```python
from build123d import *

# Parameters (mm, degrees)
F0_W     = 76.2
F0_H     = 76.2
F1_DEPTH = 76.2
F3_D     = 25.4
F4_W     = 25.4
F4_H     = 25.4
F5_DEPTH = 12.7
F6_R     = 12.7
F7_DEPTH = 12.7
F9_DEPTH = 152.4


with BuildPart() as f1:
    # F0 (on Front) → F1 (new body)
    with BuildSketch(Plane.XZ):
        with Locations((11.565426, 19.49024)):
            Rectangle(F0_W, F0_H)
    extrude(amount=F1_DEPTH)

    # F3 (through all)
    with Locations(Plane.XY.offset(57.59024)):
        with Locations((11.565426, -38.1)):
            Hole(F3_D / 2)

    # F4 (on face) → F5 (join)
    with BuildSketch(Plane(origin=(-26.534574, 0, 0), x_dir=(0, -1, 0), z_dir=(-1, 0, 0))):
        with Locations((38.1, 19.49024)):
            Rectangle(F4_W, F4_H)
    extrude(amount=F5_DEPTH)

    # F6 (on face) → F7 (join)
    with BuildSketch(Plane.XZ.offset(76.2)):
        with Locations((11.565426, 19.49024)):
            Circle(F6_R)
    extrude(amount=F7_DEPTH)

    # F8 (on face) → F9 (join)
    with BuildSketch(Plane(origin=(0, 0, 0), x_dir=(-1, 0, 0), z_dir=(0, 1, 0))):
        Polygon((0.204802, 37.538857), (-36.691747, 13.577958), (2.507274, -6.394941), align=None)
    extrude(amount=F9_DEPTH)


solid = f1.part
```
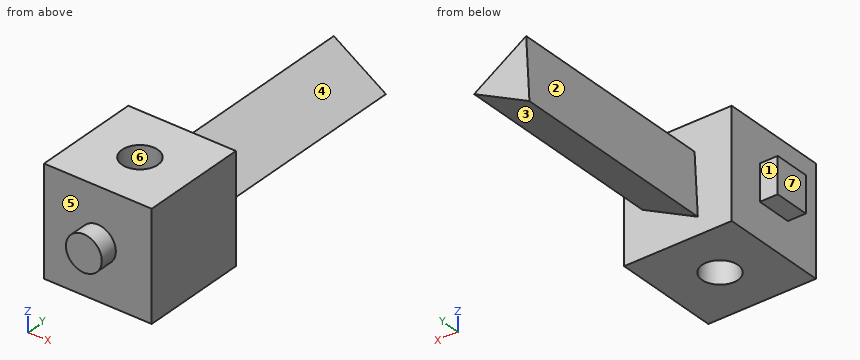
Could you check a few things on this model? Use its own coordinates, in mm. Face numbers are marked on the shaded views. A direction names the side the tool comes from. Round coordinates to 2 decimals unless told otherwise and drop trailing zeros. Write each loop counter-clockwise with the first axis right and the second up, starting at its lowest first coordinate (ties: lowest second). Pieces come first, ordered by that corner, then holes. Notation, with made-up numbers: M 13.5,-17 L 61.5,-17 A34 cw 61.5,19 Z; hole C 0,36 d9. An arc over 180 degrees is marked long. Answer in a Markdown table with one row per item. Add a question column.
Q1. If I drill on line 1 (X direction, y = -38, z = 0); line 2 (Y direction, x = -31.5, z = 12.5); line 3 (Y direction, x = -21, z = 26), over which ranges is the centre line in solid material (lowest first)? Write a range as from..to.
Q2. If we mould it in two halves opening along X, with no side actions, what happens to the marked faces 4, 5, 6 and 7? For each: +X half, -X half, draft (parallel to the pull), parting line (faces both ways), or undercut.
Q3. Imagine slicing it at D-D (y = 14). Please give me the cut outline in (x, z).
Q4. On a 3-axis mill with a long thin cutter (end or side, diameter ignored), from which of +Z, -Z, +X, -X, +Y, -Y can I reach the whole of each face in a straight line? I mean the marked faces 1, 2 and 3. Say none if no direction works.
Q5. Imagine slicing it at B-B (z = -10.5). Please give me the cut outline in (x, y), then the cut area to 3 significant figures.
Q6. Imagine slicing it at A-A (y = -38.1). Please give me the cut outline in (x, z).
Q7. Will these pins go through, and if not, where does the flat tip stop? pin 1 Ø6.5 at (x, y) = (-34, -38) entering from +Z; pin 2 Ø5 at (y, z) = (-6.5, -9) entering from -X; pin 3 Ø4 at (x, z) = (-32, 18.5) entering from -Y; pin 4 Ø10 at (x, y) = (-30.5, -40.5) entering from -Z.
Q8. Imagine slicing it at C-C (x = 42.5). Please give me the cut outline in (y, z), then the cut area to 3 significant figures.
Values:
| question | item | result |
|---|---|---|
| 1 | line 1 | -26.53..-1.13, 24.27..49.67 |
| 1 | line 2 | -50.8..-25.4 |
| 1 | line 3 | -76.2..0 |
| 2 | face 4 | +X half |
| 2 | face 5 | draft |
| 2 | face 6 | undercut |
| 2 | face 7 | -X half |
| 3 | outline | M -2.51,-6.39 L 36.69,13.58 L -0.2,37.54 Z |
| 4 | face 1 | +Z, -Z, -X, +Y |
| 4 | face 2 | +Z, -X, +Y |
| 4 | face 3 | -Z, +X, +Y |
| 5 | outline | M -26.53,-76.2 L 49.67,-76.2 L 49.67,0 L -26.53,0 Z; hole C 11.57,-38.1 d25.4 |
| 5 | area | 5,300 mm^2 |
| 6 | outline | M -39.23,6.79 L -26.53,6.79 L -26.53,-18.61 L -1.13,-18.61 L -1.13,57.59 L -26.53,57.59 L -26.53,32.19 L -39.23,32.19 Z; M 24.27,-18.61 L 49.67,-18.61 L 49.67,57.59 L 24.27,57.59 Z |
| 7 | pin 1 | z = 32.19 |
| 7 | pin 2 | x = -26.53 |
| 7 | pin 3 | y = -50.8 |
| 7 | pin 4 | z = -18.61 |
| 8 | outline | M -76.2,-18.61 L 0,-18.61 L 0,57.59 L -76.2,57.59 Z |
| 8 | area | 5,810 mm^2 |
